Design review of the part built by this model. Coordinates are the model's own, in mm. A direction names the side the tool comes from. Round coordinates to 2 decimals unless told otherwise and drop trailing zeros. Loops run counter-clockwise (first coordinate to the right, second up) from the corner with the lowest first, then second, coordinate; pieces in that order, holes last. Notation, with made-up numbers: (62, -35) - (85, -35) arc R16 ccw to (85, -8) - close; hole circle Ø6 at (9.25, 53.25). An arc over 180 degrees is marked (long way). Use one line per item in the form item = value. Start each with the question number.
(1) Machinability: for faces 1 (the cylindrical face through (-2.44, 35.58, -0.54)), 2 (the cylindrical face through (-1.58, 5.75, 1.01)), which of the approach directions +Z, -Z, +X, -X, +Y, -Y give a long, thin tool a straight path to every point of the face, cutting with its end or side? Answer none if there is none.
(2) Wall thickness on probe 1 along X at (y, z) = (32.5, 0); probe 2 along Y at (x, z) = (-1.75, -1): over which ranges is each line inside the solid? List them lowest first. Write a range as [from, to].
(3) We need section A-A, the plane z = 0. Write out the cut boundary in (x, y) (3 decimals).
(4) We need section C-C, the plane y = 47. Write out the cut boundary in (x, z), then the cut area to 3 significant figures.
(5) For pin 1 (1.5 mm diameter, centred on y = 64, z = 1, fed in from -X); pin 2 (3 mm diameter, centred on x = 1, z = 0.5, fed in from -Y); pin 3 (2 mm diameter, centred on x = -2, z = -3, fed in from +Y), all flat-tipped, find the tip position at first contact; note any pin that passes through.
(6) The part is to be moulded in two halves that separate along Y. For faces 3 (the cylindrical face through (-2.44, 2.71, -0.54)), 4 (the flat face through (0, 0, 0)), 5 (the flat face through (-2, 5.5, -1)), say which applies: released by +Y, released by -Y, zero draft, split by the parting line, or undercut.
(7) We need section D-D, the plane z = -3.75. Write out the cut boundary in (x, y), then the cut area to 3 significant figures.
(8) We need section B-B, the plane x = 0. Write out the cut boundary in (y, z) (3 decimals).
from build123d import *

# Parameters (mm, degrees)
SKETCH1_R           = 2.5
BOSS_EXTRUDE1_DEPTH = 66
SKETCH8_W           = 0.625
SKETCH8_H           = 0.5


with BuildPart() as part:
    # Sketch1 → Boss-Extrude1 (new body)
    with BuildSketch(Plane(origin=(0, 0, 0), x_dir=(1, 0, 0), z_dir=(0, 1, 0))):
        with Locations(Location((0, 0, 0), (0, 0, 270))):
            Circle(SKETCH1_R)
    extrude(amount=BOSS_EXTRUDE1_DEPTH)

    # Sketch3 → Revolve1 (revolve)
    with BuildSketch(Plane(origin=(0, 0, 0), x_dir=(0, 0, -1), z_dir=(1, 0, 0))):
        with BuildLine():
            Line((0, 66), (0, 71))
            ThreePointArc((0, 71), (3.535533906, 69.535533906), (5, 66))
            Line((5, 66), (0, 66))
        make_face()
    revolve(axis=Axis((0, 66, 0), (0, 1, 0)))

    # Sketch8 → Cut-Revolve3 (revolve, cut)
    with BuildSketch(Plane(origin=(0, 66, 0), x_dir=(0, 0, -1), z_dir=(-1, 0, 0)), mode=Mode.PRIVATE) as cut_revolve3_sk:
        with Locations((2.1875, 60.25)):
            Rectangle(SKETCH8_W, SKETCH8_H)
    revolve(cut_revolve3_sk.sketch.rotate(Axis((0, 66, 0), (0, -1, 0)), 180), axis=Axis((0, 66, 0), (0, -1, 0)), mode=Mode.SUBTRACT)


solid = part.part
Data:
q1.face_1 = -Y
q1.face_2 = none
q2.probe_1 = [-2.5, 2.5]
q2.probe_2 = [0, 5.5], [6, 70.58]
q3.outline = (-5, 66) - (-2.5, 66) - (-2.5, 6) - (-1.875, 6) - (-1.875, 5.5) - (-2.5, 5.5) - (-2.5, 0) - (2.5, 0) - (2.5, 5.5) - (1.875, 5.5) - (1.875, 6) - (2.5, 6) - (2.5, 66) - (5, 66) arc R5 ccw to start
q4.outline = circle Ø5 at (0, 0)
q4.area = 19.6 mm^2
q5.pin_1 = -2.49
q5.pin_2 = 0
q5.pin_3 = 70.27
q6.face_3 = zero draft
q6.face_4 = released by -Y
q6.face_5 = undercut
q7.outline = (-3.31, 66) - (3.31, 66) arc R3.31 ccw to start
q7.area = 17.2 mm^2
q8.outline = (0, -2.5) - (5.5, -2.5) - (5.5, -1.875) - (6, -1.875) - (6, -2.5) - (66, -2.5) - (66, -5) arc R5 ccw to (66, 5) - (66, 2.5) - (6, 2.5) - (6, 1.875) - (5.5, 1.875) - (5.5, 2.5) - (0, 2.5) - close
